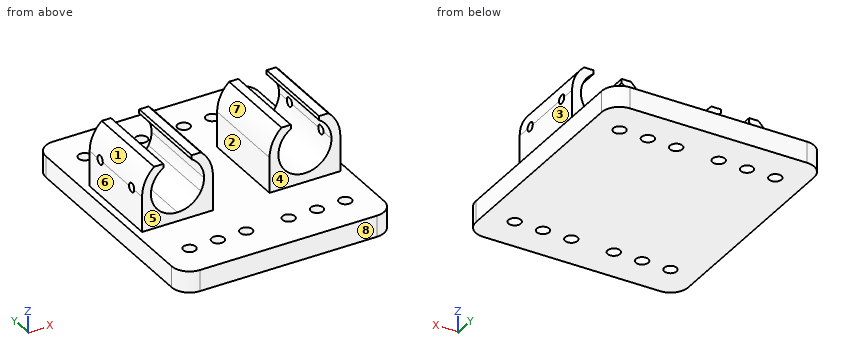
```python
from build123d import *

# Parameters (mm, degrees)
F0_W      = 60
F0_H      = 50
F0_W_2    = 20
F0_H_2    = 25
F0_H_3    = 10
F1_DEPTH  = 6
F2_DEPTH  = 10
F4_DEPTH  = 25
F5_D      = 15
F8_DEPTH  = 25
F3_R      = 7.5
F9_DEPTH  = 25
F10_R     = 5
F12_D     = 2.5
F12_DEPTH = 10
F12_START = 0.0784327
F12_TIP   = 0.7510757738
F14_D     = 2.5
F14_DEPTH = 10
F14_START = 0.0784327
F14_TIP   = 0.7510757738
F15_D     = 3.5


with BuildPart() as f1:
    # F0 (on Top) → F1 (new body)
    with BuildSketch(Plane.XY):
        Rectangle(F0_W, F0_H)
        with Locations((-18, 0)):
            Rectangle(F0_W_2, F0_H_2, mode=Mode.SUBTRACT)
        with Locations((18, 0)):
            Rectangle(F0_W_2, F0_H_2, mode=Mode.SUBTRACT)
        with Locations((0, 30)):
            Rectangle(F0_W, F0_H_3)
        with Locations((0, -30)):
            Rectangle(F0_W, F0_H_3)
        with Locations((-18, 0)):
            Rectangle(F0_W_2, F0_H_2)
        with Locations((18, 0)):
            Rectangle(F0_W_2, F0_H_2)
    extrude(amount=-F1_DEPTH)

    # F0 (on Top) → F2 (join)
    with BuildSketch(Plane.XY):
        with Locations((-18, 0)):
            Rectangle(F0_W_2, F0_H_2)
        with Locations((18, 0)):
            Rectangle(F0_W_2, F0_H_2)
    extrude(amount=F2_DEPTH)

    # F5 (through all)
    with Locations(Plane.XZ.offset(12.5)):
        with Locations((-18, 10)):
            Hole(F5_D / 2)


with BuildPart() as f4:
    # F3 (on face) → F4 (new body)
    with BuildSketch(Plane.XZ.offset(12.5)):
        with BuildLine():
            Line((-24.6143782777, 13.5355339059), (-24.6143782777, 17.5))
            ThreePointArc((-24.6143782777, 17.5), (-27.1143782777, 14.1143782777), (-28, 10))
            Line((-28, 10), (-25.5, 10))
            ThreePointArc((-25.5, 10), (-25.2752263567, 11.8223834555), (-24.6143782777, 13.5355339059))
        make_face()
        with BuildLine():
            Line((-22, 17.5), (-24.6143782777, 17.5))
            Line((-24.6143782777, 17.5), (-24.6143782777, 13.5355339059))
            ThreePointArc((-24.6143782777, 13.5355339059), (-23.4898572411, 15.1099381085), (-22, 16.3442887702))
            Line((-22, 16.3442887702), (-22, 17.5))
        make_face()
    extrude(amount=-F4_DEPTH)


with BuildPart() as f4b:
    # F3 (on face) → F4, piece 2 (new body)
    with BuildSketch(Plane.XZ.offset(12.5)):
        with BuildLine():
            Line((-11.3856217223, 13.5355339059), (-11.3856217223, 17.5))
            Line((-11.3856217223, 17.5), (-14, 17.5))
            Line((-14, 17.5), (-14, 16.3442887702))
            ThreePointArc((-14, 16.3442887702), (-12.5101427589, 15.1099381085), (-11.3856217223, 13.5355339059))
        make_face()
        with BuildLine():
            Line((-10.5, 10), (-8, 10))
            ThreePointArc((-8, 10), (-8.8856217223, 14.1143782777), (-11.3856217223, 17.5))
            Line((-11.3856217223, 17.5), (-11.3856217223, 13.5355339059))
            ThreePointArc((-11.3856217223, 13.5355339059), (-10.7247736433, 11.8223834555), (-10.5, 10))
        make_face()
    extrude(amount=-F4_DEPTH)


with BuildPart() as f1_1:
    add(f1.part)

    # F6: union F4b, F4
    add(f4b.part)
    add(f4.part)

    # F7: F1 across plane


with BuildPart() as f1_2:
    add(f1_1.part)
    add(f1_1.part.mirror(Plane.YZ))

    # F3 (on face) → F8 (cut)
    with BuildSketch(Plane.XZ.offset(12.5)):
        with BuildLine():
            ThreePointArc((-24.6143782777, 6.4644660941), (-21.8557421922, 3.5670184092), (-18, 2.5))
            ThreePointArc((-18, 2.5), (-14.1442578078, 3.5670184092), (-11.3856217223, 6.4644660941))
            Line((-11.3856217223, 6.4644660941), (-11.3856217223, 10))
            Line((-11.3856217223, 10), (-24.6143782777, 10))
            Line((-24.6143782777, 10), (-24.6143782777, 6.4644660941))
        make_face()
        with BuildLine():
            ThreePointArc((-25.5, 10), (-25.2752263567, 8.1776165445), (-24.6143782777, 6.4644660941))
            Line((-24.6143782777, 6.4644660941), (-24.6143782777, 10))
            Line((-24.6143782777, 10), (-25.5, 10))
        make_face()
        with BuildLine():
            ThreePointArc((-11.3856217223, 6.4644660941), (-10.7247736433, 8.1776165445), (-10.5, 10))
            Line((-10.5, 10), (-11.3856217223, 10))
            Line((-11.3856217223, 10), (-11.3856217223, 6.4644660941))
        make_face()
    extrude(amount=-F8_DEPTH, mode=Mode.SUBTRACT)

    # F3 (on face) → F9 (cut)
    with BuildSketch(Plane.XZ.offset(12.5)):
        with Locations((18, 10)):
            Circle(F3_R)
    extrude(amount=-F9_DEPTH, mode=Mode.SUBTRACT)

    # F10
    f10_edges = [f1_2.edges().sort_by_distance(p)[0] for p in [
        (-30, -35, -3),
        (30, -35, -3),
        (30, 35, -3),
        (-30, 35, -3),
    ]]
    fillet(f10_edges, radius=F10_R)

    # F12
    # its depths count from where the whole tool has entered the part; down to there all is cleared
    with Locations(Plane.YZ.offset(28).offset(-F12_START)):
        with Locations((-7.5, 10), (7.5, 10)):
            Hole(F12_D / 2, depth=F12_DEPTH)
            with Locations((0, 0, -(F12_DEPTH + F12_TIP / 2))):  # 118° drill point
                Cone(0, F12_D / 2, F12_TIP, mode=Mode.SUBTRACT)

    # F14
    # its depths count from where the whole tool has entered the part; down to there all is cleared
    with Locations(Plane(origin=(-28, 0, 0), x_dir=(0, -1, 0), z_dir=(-1, 0, 0)).offset(-F14_START)):
        with Locations((-7.5, 10), (7.5, 10)):
            Hole(F14_D / 2, depth=F14_DEPTH)
            with Locations((0, 0, -(F14_DEPTH + F14_TIP / 2))):  # 118° drill point
                Cone(0, F14_D / 2, F14_TIP, mode=Mode.SUBTRACT)

    # F15 (through all)
    with Locations(Plane.XY):
        with Locations((-22, -25), (-14, -25), (-6, -25), (6, -25), (14, -25), (22, -25), (-22, 25), (-14, 25), (-6, 25), (6, 25), (14, 25), (22, 25)):
            Hole(F15_D / 2)


solid = f1_2.part
```
Model file for the job. Use its own axes, mm. Face numbers are marked on the shaded views. A direction names the side the tool comes from. Coordinates: 2 decimals unless noted, no trailing zeros. Order: outer loops, then holes, each group sorted by start corner. A loop starts at its lowest first (then second) coordinate and runs counter-clockwise, first axis right, second up. Notation, with made-up numbers: (45, 64) -> (58, 64) arc R24 ccw to (58, 93) -> close; hole circle Ø3 at (-18.75, 49). An arc over 180 degrees is marked (long way). Return JSON: item names as keys, results as strings.
Item 1: Slice it at C-C (y = -25). Write the cut outline in (x, z).
Model answer:
{"outline": "(-30, -6) -> (-23.75, -6) -> (-23.75, 0) -> (-30, 0) -> close; (-20.25, -6) -> (-15.75, -6) -> (-15.75, 0) -> (-20.25, 0) -> close; (-12.25, -6) -> (-7.75, -6) -> (-7.75, 0) -> (-12.25, 0) -> close; (-4.25, -6) -> (4.25, -6) -> (4.25, 0) -> (-4.25, 0) -> close; (7.75, -6) -> (12.25, -6) -> (12.25, 0) -> (7.75, 0) -> close; (15.75, -6) -> (20.25, -6) -> (20.25, 0) -> (15.75, 0) -> close; (23.75, -6) -> (30, -6) -> (30, 0) -> (23.75, 0) -> close"}
Item 2: Slice it at D-D (z = 7.5). Write the cut outline in (x, y).
Model answer:
{"outline": "(-28, -12.5) -> (-25.07, -12.5) -> (-25.07, 12.5) -> (-28, 12.5) -> close; (-10.93, -12.5) -> (-8, -12.5) -> (-8, 12.5) -> (-10.93, 12.5) -> close; (8, -12.5) -> (10.93, -12.5) -> (10.93, 12.5) -> (8, 12.5) -> close; (25.07, -12.5) -> (28, -12.5) -> (28, 12.5) -> (25.07, 12.5) -> close"}
Item 3: Wall check: line 1 along Y through (x, z) = (27.25, 10); line 2 along Y through (x, z) = (22, -2.1); line 3 along X through (y, z) = (4, 12.75). Give the ranges that are in metal, low to high. Write a range as from..to.
Model answer:
{"line 1": "y = -12.5..-8.75, -6.25..6.25, 8.75..12.5", "line 2": "y = -35..-26.75, -23.25..23.25, 26.75..35", "line 3": "x = -27.61..-24.98, -11.02..-8.39, 8.39..11.02, 24.98..27.61"}
Item 4: Pin check, flat tips, straight feed: P1, Ø1, axis at x = 24, y = 20.5, coming from the +Z side; P2, Ø11, axis at y = 3, z = 6.5, coming from the -X side; P3, Ø3, axis at x = -22, y = 25, coming from the -Z side; P4, Ø8, axis at x = 4.5, z = 8.5, coming from the +Y side. Stop position of each tip, or through.
Model answer:
{"P1": "stops at z = 0", "P2": "stops at x = -28", "P3": "passes through", "P4": "stops at y = 12.5"}
Item 5: Slice it at B-B (x = -6). Write the cut outline in (y, z).
Model answer:
{"outline": "(-35, -6) -> (-26.75, -6) -> (-26.75, 0) -> (-35, 0) -> close; (-23.25, -6) -> (23.25, -6) -> (23.25, 0) -> (-23.25, 0) -> close; (26.75, -6) -> (35, -6) -> (35, 0) -> (26.75, 0) -> close"}
Item 6: 3-axis set-ups, long thin cutter, end or side, ignore diameter. For the marked faces 5, 6, 7 and 8: which of +Z, -Z, +X, -X, +Y, -Y reach the whole face in a straight line?
Model answer:
{"face 5": "+Z, +X, -X, -Y", "face 6": "+Z, -X, +Y, -Y", "face 7": "+Z, +Y, -Y", "face 8": "+Z, -Z, +X, -X, -Y"}
Item 7: Mould opens along X. For the marked faces 1, 2, 3 and 4 say: pulls with the +X half, pulls with the -X half, needs draft (parallel to the pull), parting line crosses it, or undercut.
Model answer:
{"face 1": "pulls with the -X half", "face 2": "undercut", "face 3": "pulls with the +X half", "face 4": "needs draft"}
Item 8: Slice it at A-A (z = -1.75). Count the separate pieces of the cut face and the enclosed holes in it, then the cut area to 3 significant figures.
Model answer:
{"separate pieces": "1", "enclosed holes": "12", "area": "4,060 mm²"}
